from build123d import *

# Parameters (mm, degrees)
F0_W     = 19.07
F0_H     = 10.5
F1_DEPTH = 10.5
F2_R     = 3.525
F3_DEPTH = 10.5
F5_DEPTH = 10.5


with BuildPart() as f1:
    # F0 (on Front) → F1 (new body)
    with BuildSketch(Plane.XZ):
        Rectangle(F0_W, F0_H)
    extrude(amount=-F1_DEPTH)

    # F2 (on face) → F3 (cut, through all)
    with BuildSketch(Plane.XZ):
        with BuildLine():
            ThreePointArc((-4.285, -5.25), (-7.997311, -3.712311), (-9.535, 0))
            Line((-9.535, 0), (-9.535, -5.25))
            Line((-9.535, -5.25), (-4.285, -5.25))
        make_face()
        with BuildLine():
            ThreePointArc((-9.535, 0), (-7.997311, 3.712311), (-4.285, 5.25))
            Line((-4.285, 5.25), (-9.535, 5.25))
            Line((-9.535, 5.25), (-9.535, 0))
        make_face()
        with Locations((-4.285, 0)):
            Circle(F2_R)
    extrude(amount=-F3_DEPTH, mode=Mode.SUBTRACT)

    # F4 (on face) → F5 (cut, through all)
    with BuildSketch(Plane.XY.offset(5.25)):
        with BuildLine():
            ThreePointArc((6.035, 0.300253), (5.172785, 0.075608), (4.285, 0))
            Line((4.285, 0), (9.535, 0))
            Line((9.535, 0), (9.535, 10.5))
            Line((9.535, 10.5), (4.285, 10.5))
            ThreePointArc((4.285, 10.5), (5.172785, 10.424392), (6.035, 10.199747))
            Line((6.035, 10.199747), (6.035, 8.309922))
            ThreePointArc((6.035, 8.309922), (0.76, 5.25), (6.035, 2.190078))
            Line((6.035, 2.190078), (6.035, 0.300253))
        make_face()
    extrude(amount=-F5_DEPTH, mode=Mode.SUBTRACT)


solid = f1.part
Input: part model. Units: mm. Frame: model coordinates. Coordinates: 2 decimals unless noted, no trailing zeros. Write each loop counter-clockwise with the first axis right and the second up, starting at its lowest first coordinate (ties: lowest second). Pieces come first, ordered by that corner, then holes. Notation, with made-up numbers: M 57.5,56.5 L 115.5,56.5 A33 cw 115.5,93.5 Z; hole C 32.5,60.25 d7. An arc over 180 degrees is marked long. Answer as a JSON object with one key per item and string values. Group by question number.
(1) Section B-B on y = 9.75. Output: boundary loops of the cut face in (x, z) (3 decimals).
(2) Section A-A on x = 4.75. Output: boundary loops of the cut face in (y, z).
(3) Ray query, line 1 along Y through (x, z) = (4.25, 3.25); line 2 along Z through (x, y) = (-4.5, 8.25); line 3 along X through (y, z) = (5.5, 2). Return the intervals inside material, ascending. Write a range as [from, to].
(4) Mould query, pull axis Y, two halves, no side actions, for faces 1 (the face through (5.19, 0.08, 0.07)), 2 (the face through (0.76, 5.35, 0.07)), 3 (the face through (0, 5, 5.25)). Classes: pulls with the +Y half, pulls with the -Y half, needs draft (parallel to the pull), parting line crosses it, or undercut.
(5) Section D-D on x = -7. Output: boundary loops of the cut face in (y, z).
(6) Section C-C on z = 1.5. Output: boundary loops of the cut face in (x, y) (3 decimals), plus the area to 3 significant figures.
(7) Contact query for flat-ended pins moving along their axis: P1, Ø4, axis at y = 5, z = 3, coming from the +X side; P2, Ø4, axis at y = 3.5, z = 3, coming from the -X side; P3, Ø1, axis at y = 6.5, z = 4, coming from the -X side. Output: stop coordinate, or through.
Result set:
{
 "1": {"outline": "M -9.535,0 A5.25 ccw -4.285,-5.25 L 6.035,-5.25 L 6.035,5.25 L -4.285,5.25 A5.25 ccw Z; hole C -4.285,0 d7.05"},
 "2": {"outline": "M 0.02,-5.25 L 1.76,-5.25 L 1.76,5.25 L 0.02,5.25 Z; M 8.74,-5.25 L 10.48,-5.25 L 10.48,5.25 L 8.74,5.25 Z"},
 "3": {"line 1": "y = [0, 1.73], [8.77, 10.5]", "line 2": "z = [-5.25, -3.52], [3.52, 5.25]", "line 3": "x = [-9.14, -7.19], [-1.38, 0.77]"},
 "4": {"face 1": "pulls with the -Y half", "face 2": "undercut", "face 3": "needs draft"},
 "5": {"outline": "M 0,-4.49 L 10.5,-4.49 L 10.5,-2.25 L 0,-2.25 Z; M 0,2.25 L 10.5,2.25 L 10.5,4.49 L 0,4.49 Z"},
 "6": {"outline": "M -9.316,0 L -7.475,0 L -7.475,10.5 L -9.316,10.5 Z; M -1.095,0 L 4.285,0 A5.25 ccw 6.035,0.3 L 6.035,2.19 A3.525 cw long 6.035,8.31 L 6.035,10.2 A5.25 ccw 4.285,10.5 L -1.095,10.5 Z", "area": "62.5 mm2"},
 "7": {"P1": "stops at x = 1.57", "P2": "stops at x = -9.44", "P3": "stops at x = -8.2"}
}
